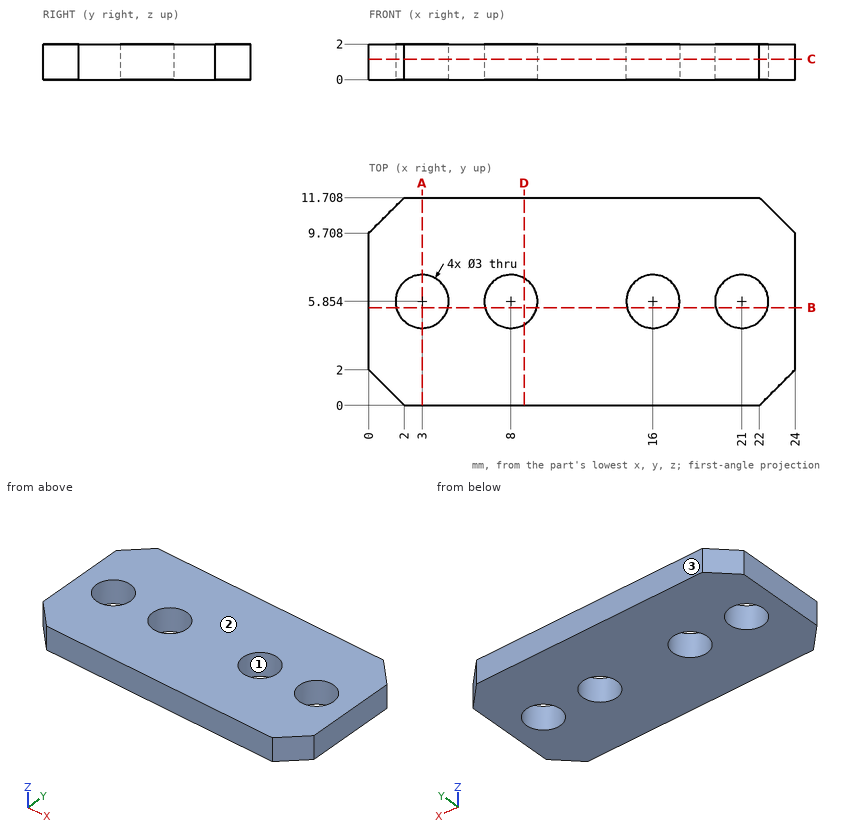
Can you work these out from the drawing? Everything is in mm from the part's minimum corner. Coordinates: 2 decimals unless noted, no trailing zeros. Loops run counter-clockwise (first coordinate to the right, second up) from the corner with the lowest first, then second, coordinate; pieces in that order, holes last. Notation, with made-up numbers: (32.5, 53) - (45.5, 53) arc R29 cw to (45.5, 89) - close; hole circle Ø8 at (82.25, 74). An arc over 180 degrees is marked (long way). Use a Markdown table: item, result.
Item 1: I want a section at C-C on z = 1.15. Please give me the cut outline in (x, y) (1 decimal).
Numbers:
| item | result |
|---|---|
| outline | (0, 2) - (2, 0) - (22, 0) - (24, 2) - (24, 9.7) - (22, 11.7) - (2, 11.7) - (0, 9.7) - close; hole circle Ø3 at (3, 5.9); hole circle Ø3 at (8, 5.9); hole circle Ø3 at (16, 5.9); hole circle Ø3 at (21, 5.9) |
Item 2: We'd pull the mould along Y, two halves only. Please class the marked faces 1, 2 and 3: released by +Y, released by -Y, zero draft, split by the parting line, or undercut.
Numbers:
| item | result |
|---|---|
| face 1 | undercut |
| face 2 | zero draft |
| face 3 | released by +Y |
Item 3: I want a section at D-D on x = 8.75. Please give me the cut outline in (y, z) (1 decimal).
Numbers:
| item | result |
|---|---|
| outline | (0, 0) - (4.6, 0) - (4.6, 2) - (0, 2) - close; (7.2, 0) - (11.7, 0) - (11.7, 2) - (7.2, 2) - close |
Item 4: I want a section at A-A on x = 3. Please give me the cut outline in (y, z) (1 decimal).
Numbers:
| item | result |
|---|---|
| outline | (0, 0) - (4.4, 0) - (4.4, 2) - (0, 2) - close; (7.4, 0) - (11.7, 0) - (11.7, 2) - (7.4, 2) - close |
Item 5: Will this pin go through, and if not, where does the flat tip stop? pin 1 (1.8 mm diameter, centred on x = 3, y = 5.85, fed in from +Z).
Numbers:
| item | result |
|---|---|
| pin 1 | passes through |
Item 6: If I drill on probe 1 along X at (y, z) = (5.75, 0.55); probe 2 along Y at (x, z) = (3, 0.7) (1 decimal); probe 3 along X at (y, z) = (5, 0.1) (1 decimal), over which ranges is the centre line in solid material (lowest first)? Write a range as from..to.
Numbers:
| item | result |
|---|---|
| probe 1 | x = 0..1.5, 4.5..6.5, 9.5..14.5, 17.5..19.5, 22.5..24 |
| probe 2 | y = 0..4.4, 7.4..11.7 |
| probe 3 | x = 0..1.8, 4.2..6.8, 9.2..14.8, 17.2..19.8, 22.2..24 |
Item 7: I want a section at B-B on y = 5.5. Please give me the cut outline in (x, z).
Numbers:
| item | result |
|---|---|
| outline | (0, 0) - (1.54, 0) - (1.54, 2) - (0, 2) - close; (4.46, 0) - (6.54, 0) - (6.54, 2) - (4.46, 2) - close; (9.46, 0) - (14.54, 0) - (14.54, 2) - (9.46, 2) - close; (17.46, 0) - (19.54, 0) - (19.54, 2) - (17.46, 2) - close; (22.46, 0) - (24, 0) - (24, 2) - (22.46, 2) - close |
